Could you check a few things on this drawing? It's one solid part, dimensions in mm from its lowest x, y, z. A direction names the side the tool comes from. Coordinates: 2 decimals unless noted, no trailing zeros. Loops run counter-clockwise (first coordinate to the right, second up) from the corner with the lowest first, then second, coordinate; pieces in that order, holes last. Notation, with made-up numbers: (-27.75, -26.75) -> (-2.75, -26.75) arc R24 ccw to (-2.75, -5.75) -> close; hole circle Ø1 at (85.5, -25). An arc over 180 degrees is marked (long way). One line per question, with ' | ' between items.
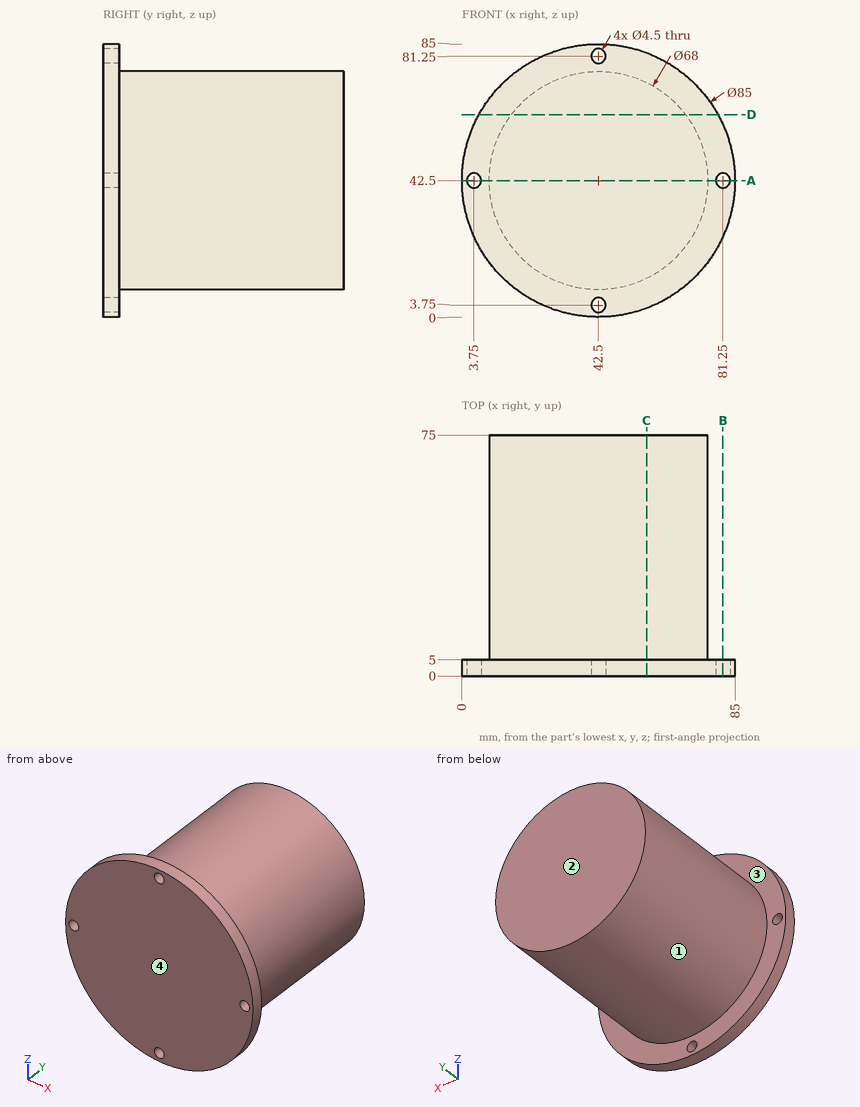
1) If we section it at D-D on z = 63: Please give me the cut outline in (x, y), and give its area (3 significant figures).
Data:
outline: (5.27, 0) -> (79.73, 0) -> (79.73, 5) -> (69.62, 5) -> (69.62, 75) -> (15.38, 75) -> (15.38, 5) -> (5.27, 5) -> close | area: 4,170 mm²
2) If we section it at C-C on x = 57.5: Please give me the cut outline in (y, z), and give its area (3 significant figures).
Data:
outline: (0, 2.74) -> (5, 2.74) -> (5, 11.99) -> (75, 11.99) -> (75, 73.01) -> (5, 73.01) -> (5, 82.26) -> (0, 82.26) -> close | area: 4,670 mm²
3) I need wall thicknesses on line 1 along Z through (x, y) = (42, 1); line 2 along Y through (x, z) = (55, 10); line 3 along X through (y, z) = (40, 43). Which ranges of each line are inside material? Lowest first, please. Write a range as from..to.
Data:
line 1: 0..1.56, 5.94..79.06, 83.44..85 | line 2: 0..5 | line 3: 8.5..76.5
4) On a 3-axis mill with a long thin cutter (end or side, diameter ignored), from which of +Z, -Z, +X, -X, +Y, -Y can I reach the whole of each face in a straight line? I mean the marked faces 3 and 4. Say none if no direction works.
Data:
face 3: +Y | face 4: +Z, -Z, +X, -X, -Y
5) I'm going to push flat-ended pins straight in: pin 1 Ø12 at (x, y) = (64, 42.5) entering from +Z; pin 2 Ø8 at (y, z) = (35, 57) entering from +X; pin 3 Ø4 at (x, y) = (65.5, 19) entering from +Z; pin 4 Ø4 at (x, z) = (32, 19.5) entering from -Y. Where does each tip first touch, or does it pass through?
Data:
pin 1: z = 72.76 | pin 2: x = 74.84 | pin 3: z = 69.24 | pin 4: y = 0
6) We'd pull the mould along Z, two halves only. Please class the marked faces 1 and 2: pulls with the +Z half, pulls with the -Z half, needs draft (parallel to the pull), parting line crosses it, or undercut.
Data:
face 1: parting line crosses it | face 2: needs draft
7) If we section it at A-A on z = 42.5: Please give me the cut outline in (x, y).
Data:
outline: (0, 0) -> (1.5, 0) -> (1.5, 5) -> (0, 5) -> close; (6, 0) -> (79, 0) -> (79, 5) -> (76.5, 5) -> (76.5, 75) -> (8.5, 75) -> (8.5, 5) -> (6, 5) -> close; (83.5, 0) -> (85, 0) -> (85, 5) -> (83.5, 5) -> close
8) If we section it at B-B on x = 81.25: Please give me the cut outline in (y, z).
Data:
outline: (0, 25.04) -> (5, 25.04) -> (5, 40.25) -> (0, 40.25) -> close; (0, 44.75) -> (5, 44.75) -> (5, 59.96) -> (0, 59.96) -> close
